Can you work these out from the model? Positions are in its coordinate system, mm. Face numbers are marked on the shaded views. A direction names the side the tool comes from. Round coordinates to 2 decimals unless told otherwise and drop trailing zeros. Order: outer loops, then holes, each group sorted by start corner. A loop starts at its lowest first (then second) coordinate and runs counter-clockwise, first axis right, second up. Notation, with made-up numbers: M 23,-10 L 71,-10 A21 ccw 71,27 Z; hole C 76,21.25 d3. An arc over 180 degrees is marked long. One line per question, with ' | ' between items.
```python
from build123d import *

# Parameters (mm, degrees)
F0_R      = 6.05
F1_DEPTH  = 20
F3_DEPTH  = 25
F4_W      = 5.75
F4_H      = 2.75
F5_DEPTH  = 7.5
F6_R      = 1.55
F7_DEPTH  = 10
F9_R      = 1.5
F10_DEPTH = 10


with BuildPart() as f1:
    # F0 (on Front) → F1 (new body)
    with BuildSketch(Plane.XZ):
        with BuildLine():
            Line((-6, 18), (-6, 8))
            ThreePointArc((-6, 8), (0, -10), (6, 8))
            Line((6, 8), (6, 18))
            Line((6, 18), (-6, 18))
        make_face()
        Circle(F0_R, mode=Mode.SUBTRACT)
    extrude(amount=F1_DEPTH)

    # F2 (on face) → F3 (cut)
    with BuildSketch(Plane.YZ.offset(6)):
        with BuildLine():
            Line((0, 12.5), (-7.04196, 12.5))
            ThreePointArc((-7.04196, 12.5), (-13, 12), (-7.04196, 11.5))
            Line((-7.04196, 11.5), (0, 11.5))
            Line((0, 11.5), (0, 12.5))
        make_face()
    extrude(amount=-F3_DEPTH, mode=Mode.SUBTRACT)

    # F4 (on face) → F5 (cut)
    with BuildSketch(Plane(origin=(0, 0, 0), x_dir=(-1, 0, 0), z_dir=(0, 1, 0))):
        with Locations((0, 8.625)):
            Rectangle(F4_W, F4_H)
    extrude(amount=-F5_DEPTH, mode=Mode.SUBTRACT)

    # F6 (on face) → F7 (cut)
    with BuildSketch(Plane.XY.offset(18)):
        with Locations((0, -4)):
            Circle(F6_R)
    extrude(amount=-F7_DEPTH, mode=Mode.SUBTRACT)

    # F9 (on face) → F10 (cut)
    with BuildSketch(Plane.XY.offset(18)):
        with Locations((-3, -16.5)):
            Circle(F9_R)
        with Locations((3, -16.5)):
            Circle(F9_R)
    extrude(amount=-F10_DEPTH, mode=Mode.SUBTRACT)


solid = f1.part
```
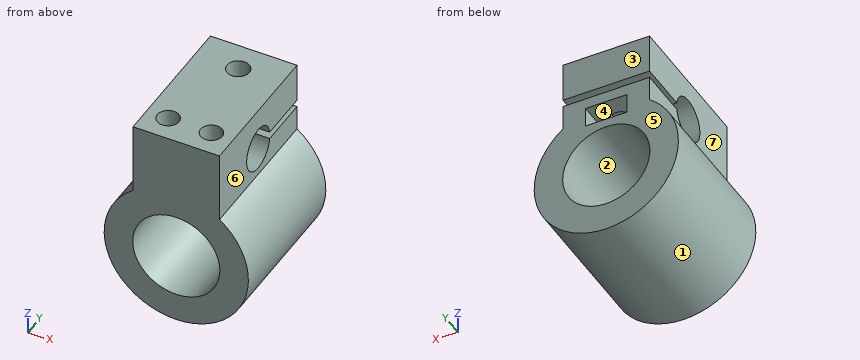
(1) If we section it at A-A on y = -1.5: Please give me the cut outline in (x, z) (3 decimals), plus the area to 3 significant figures.
Final values:
outline: M -6,8 A10 ccw long 6,8 L 6,11.5 L -6,11.5 Z; M -6,12.5 L 6,12.5 L 6,18 L -6,18 Z; hole C 0,0 d12.1; hole M -2.875,7.25 L 2.875,7.25 L 2.875,10 L -2.875,10 Z | area: 275 mm^2
(2) Will these pins go through, and if not, where does the flat tip stop? pin 1 Ø2 at (y, z) = (-3.5, 8) entering from +X; pin 2 Ø3 at (x, y) = (0, -4) entering from +Z; pin 3 Ø6 at (y, z) = (-16, 6) entering from -X.
Final values:
pin 1: x = 7.14 | pin 2: z = 7.25 | pin 3: x = -9.54
(3) If we section it at C-C on z = 0: Please give me the cut outline in (x, y), plus the area to 3 significant figures.
Final values:
outline: M -10,-20 L -6.05,-20 L -6.05,0 L -10,0 Z; M 6.05,-20 L 10,-20 L 10,0 L 6.05,0 Z | area: 158 mm^2
(4) Please list where these lines run through material, in increasing order: probe 1 along Z at (x, y) = (0, -10); probe 2 along Z at (x, y) = (0, -12.25); probe 3 along Y at (x, z) = (-0.75, 13.25). Write a range as [from, to].
Final values:
probe 1: [-10, -6.05], [6.05, 9], [15, 18] | probe 2: [-10, -6.05], [6.05, 10.02], [13.98, 18] | probe 3: [-20, -12.73], [-7.27, -5.36], [-2.64, 0]
(5) On a 3-axis mill with a long thin cutter (end or side, diameter ignored), from which of +Z, -Z, +X, -X, +Y, -Y can I reach the whole of each face in a straight line? I mean the marked faces 5, 6 and 7. Say none if no direction works.
Final values:
face 5: +Z, -Z, +X, -X, +Y | face 6: +Z, +X, +Y, -Y | face 7: +Z, -X, +Y, -Y
(6) If we section it at B-B on y = -4: Please give me the cut outline in (x, z) (3 decimals).
Final values:
outline: M -6,8 A10 ccw long 6,8 L 6,11.5 L 1.55,11.5 L 1.55,10 L 2.875,10 L 2.875,7.25 L -2.875,7.25 L -2.875,10 L -1.55,10 L -1.55,11.5 L -6,11.5 Z; M -6,12.5 L -1.55,12.5 L -1.55,18 L -6,18 Z; M 1.55,12.5 L 6,12.5 L 6,18 L 1.55,18 Z; hole C 0,0 d12.1
(7) Thinking about a two-plate mould opening in Z: for the marked faces 1, 2, 3 and 4, which applies, released by +Z, released by -Z, zero draft, split by the parting line, or undercut?
Final values:
face 1: split by the parting line | face 2: undercut | face 3: zero draft | face 4: undercut
(8) If we section it at D-D on x = 0: Please give me the cut outline in (y, z).
Final values:
outline: M -20,-10 L 0,-10 L 0,-6.05 L -20,-6.05 Z; M -20,6.05 L 0,6.05 L 0,7.25 L -7.5,7.25 L -7.5,10 L -5.55,10 L -5.55,11.5 L -7.04,11.5 A3 cw long -7.04,12.5 L -5.55,12.5 L -5.55,18 L -20,18 Z; M -2.45,10 L 0,10 L 0,11.5 L -2.45,11.5 Z; M -2.45,12.5 L 0,12.5 L 0,18 L -2.45,18 Z
